```python
from build123d import *

# Parameters (mm, degrees)
SKETCH1_R                = 33
SKETCH1_R_2              = 29.5
BOSS_EXTRUDE1_DEPTH      = 6
SKETCH2_R                = 33
SKETCH2_R_2              = 2
BOSS_EXTRUDE2_DEPTH      = 1
SKETCH3_R                = 6.25
CUT_EXTRUDE2_DEPTH       = 7
CIRPATTERN1_COUNT        = 6
BOSS_EXTRUDE3_DEPTH      = 1.25
BOSS_EXTRUDE3_DEPTH_BACK = 7.25
SKETCH4_R                = 35.5
SKETCH4_R_2              = 31.5


with BuildPart() as part:
    # Sketch1 → Boss-Extrude1 (new body)
    with BuildSketch(Plane.XY):
        Circle(SKETCH1_R)
        Circle(SKETCH1_R_2, mode=Mode.SUBTRACT)
    extrude(amount=BOSS_EXTRUDE1_DEPTH)

    # Sketch2 → Boss-Extrude2 (add)
    with BuildSketch(Plane(origin=(0, 0, 0), x_dir=(-1, 0, 0), z_dir=(0, 0, -1))):
        with Locations(Location((0, 0, 0), (0, 0, 180))):
            Circle(SKETCH2_R)
        Circle(SKETCH2_R_2, mode=Mode.SUBTRACT)
    extrude(amount=-BOSS_EXTRUDE2_DEPTH)

    # Sketch3 → Cut-Extrude2 (cut)
    with BuildSketch(Plane(origin=(0, 0, 0), x_dir=(-1, 0, 0), z_dir=(0, 0, -1))):
        with Locations((1.444237573, -18.192764436)):
            Circle(SKETCH3_R)
    cut_extrude2 = extrude(amount=-CUT_EXTRUDE2_DEPTH, mode=Mode.SUBTRACT)

    # CirPattern1: Cut-Extrude2 ×6 about axis
    cirpattern1_axis = Axis((0, 0, 0), (0, 0, 1))
    for i in range(1, CIRPATTERN1_COUNT):
        add(cut_extrude2.rotate(cirpattern1_axis, i * 360 / CIRPATTERN1_COUNT), mode=Mode.SUBTRACT)

    # Sketch4 → Boss-Extrude3 (add, two sides: drawn at the far end of the back side and taken through both)
    with BuildSketch(Plane(origin=(0, 0, 0), x_dir=(-1, 0, 0), z_dir=(0, 0, -1)).offset(-BOSS_EXTRUDE3_DEPTH_BACK)):
        Circle(SKETCH4_R)
        with Locations(Location((0, 0, 0), (0, 0, 180))):
            Circle(SKETCH4_R_2, mode=Mode.SUBTRACT)
    extrude(amount=BOSS_EXTRUDE3_DEPTH + BOSS_EXTRUDE3_DEPTH_BACK)


solid = part.part
```
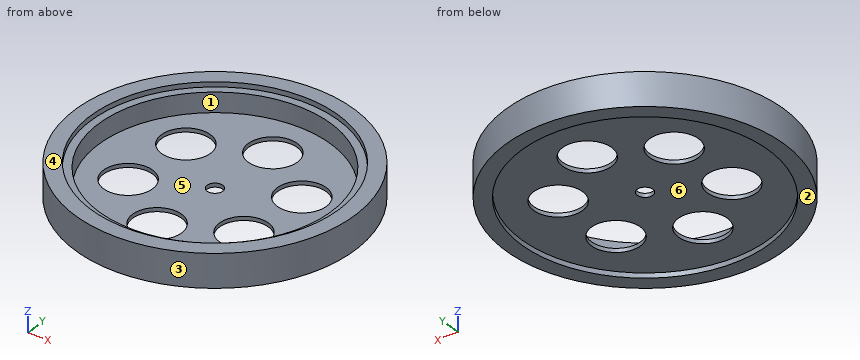
The model under review builds one solid part; all positions refer to its coordinate system, in mm. Face numbers are marked on the shaded views. A direction names the side the tool comes from. Round coordinates to 2 decimals unless told otherwise and drop trailing zeros. Order: outer loops, then holes, each group sorted by start corner. A loop starts at its lowest first (then second) coordinate and runs counter-clockwise, first axis right, second up.
(1) For P1, Ø3, axis at x = 12.5, y = 15, coming from the +Z side; P2, Ø1.5, axis at x = -22.5, y = -15.5, coming from the -Z side; P3, Ø10, axis at x = 16.48, y = 7.85, coming from the +Z side; P4, Ø1, axis at y = -6.5, z = 0.5, coming from the -X side, all flat-tipped, find the tip position at first contact; note any pin that passes through.
Working result:
P1: stops at z = 1
P2: stops at z = 0
P3: passes through
P4: stops at x = -34.99
(2) Mouldability with a two-part tool opening along Y and no side actions: class the marked faces 3, 4, 5 and 6 as released by +Y, released by -Y, zero draft, split by the parting line, or undercut.
Working result:
face 3: split by the parting line
face 4: zero draft
face 5: undercut
face 6: undercut
(3) Wall thickness on L1, parallel to Y at x = 0, z = -0.9; L2, parallel to X at y = -1, z = 5.75; L3, parallel to Y at x = 4, z = 0.25: over which ranges is each line inside the solid? List them lowest first.
Working result:
L1: y = -35.5 to -31.5, 31.5 to 35.5
L2: x = -35.49 to -29.48, 29.48 to 35.49
L3: y = -35.27 to -21.26, -15.12 to 12.49, 23.9 to 35.27
(4) Take a section at C-C, the plane y = -20. State the section outline as (x, z) points.
Working result:
outline: (-29.33, -1.25) - (-24.34, -1.25) - (-24.34, 0) - (-7.43, 0) - (-7.43, 1) - (-21.69, 1) - (-21.69, 6) - (-24.34, 6) - (-24.34, 7.25) - (-29.33, 7.25) - close; (4.54, 0) - (24.34, 0) - (24.34, -1.25) - (29.33, -1.25) - (29.33, 7.25) - (24.34, 7.25) - (24.34, 6) - (21.69, 6) - (21.69, 1) - (4.54, 1) - close
(5) Take a section at D-D, the plane x = 27.5. State the section outline as (y, z) points.
Working result:
outline: (-22.45, -1.25) - (-15.36, -1.25) - (-15.36, 0) - (15.36, 0) - (15.36, -1.25) - (22.45, -1.25) - (22.45, 7.25) - (15.36, 7.25) - (15.36, 6) - (10.68, 6) - (10.68, 1) - (-10.68, 1) - (-10.68, 6) - (-15.36, 6) - (-15.36, 7.25) - (-22.45, 7.25) - close
(6) Take a section at A-A, the plane y = 0. State the section outline as (x, z) points, plus the area to 3 significant figures.
Working result:
outline: (-35.5, -1.25) - (-31.5, -1.25) - (-31.5, 0) - (-2, 0) - (-2, 1) - (-29.5, 1) - (-29.5, 6) - (-31.5, 6) - (-31.5, 7.25) - (-35.5, 7.25) - close; (2, 0) - (31.5, 0) - (31.5, -1.25) - (35.5, -1.25) - (35.5, 7.25) - (31.5, 7.25) - (31.5, 6) - (29.5, 6) - (29.5, 1) - (2, 1) - close
area: 147 mm2
(7) Tool access review of the marked faces 1 and 2: name each direction out of +Z, -Z, +X, -X, +Y, -Y from which nothing blocks a thin tool from reaching the whole face with its end or side.
Working result:
face 1: +Z
face 2: -Z, +X, -X, +Y, -Y
(8) Take a section at B-B, the plane x = 0. State the section outline as (y, z) points, plus the area to 3 significant figures.
Working result:
outline: (-35.5, -1.25) - (-31.5, -1.25) - (-31.5, 0) - (-24.27, 0) - (-24.27, 1) - (-29.5, 1) - (-29.5, 6) - (-31.5, 6) - (-31.5, 7.25) - (-35.5, 7.25) - close; (-12.11, 0) - (-2, 0) - (-2, 1) - (-12.11, 1) - close; (2, 0) - (12.11, 0) - (12.11, 1) - (2, 1) - close; (24.27, 0) - (31.5, 0) - (31.5, -1.25) - (35.5, -1.25) - (35.5, 7.25) - (31.5, 7.25) - (31.5, 6) - (29.5, 6) - (29.5, 1) - (24.27, 1) - close
area: 123 mm2
